Work out the finished part from the listing and answer in its coordinate system (mm). Round coordinates to 2 decimals unless told otherwise and drop trailing zeros. Write each loop counter-clockwise with the first axis right and the second up, starting at its lowest first coordinate (ties: lowest second). Pieces come first, ordered by that corner, then holes. Notation, with made-up numbers: (-1.5, 53) - (47.5, 53) arc R32 ccw to (47.5, 80) - close; hole circle Ø6 at (15.25, 45.5). An arc over 180 degrees is marked (long way). Answer as a JSON object with one key per item and string values.
```python
from build123d import *

# Parameters (mm, degrees)
BOSS_EXTRUDE1_DEPTH = 774.7
SKETCH2_W           = 344.402501539
SKETCH2_H           = 780.457540957
CUT_EXTRUDE1_DEPTH  = 59.371664787


with BuildPart() as part:
    # Sketch1 → Boss-Extrude1 (new body)
    with BuildSketch(Plane(origin=(0, 0, 0), x_dir=(0, 0, -1), z_dir=(1, 0, 0))):
        with BuildLine():
            Line((0, 0), (31.75, 0))
            ThreePointArc((31.75, 0), (54.200640303, 9.299359697), (63.5, 31.75))
            Line((63.5, 31.75), (63.5, 95.25))
            ThreePointArc((63.5, 95.25), (54.200640303, 117.700640303), (31.75, 127))
            Line((31.75, 127), (0, 127))
            Line((0, 127), (-19.05, 127))
            Line((-19.05, 127), (-19.05, 0))
            Line((-19.05, 0), (0, 0))
        make_face()
    extrude(amount=BOSS_EXTRUDE1_DEPTH)

    # Sketch2 → Cut-Extrude1 (cut, through all)
    with BuildSketch(Plane(origin=(355.6, 0, 355.6), x_dir=(0, 1, 0), z_dir=(0.707106781, 0, 0.707106781))):
        with Locations((32.995160032, -592.696903991)):
            Rectangle(SKETCH2_W, SKETCH2_H)
    cut_extrude1 = extrude(amount=CUT_EXTRUDE1_DEPTH, mode=Mode.SUBTRACT)

    # Mirror1: Cut-Extrude1 across plane
    add(cut_extrude1.mirror(Plane(origin=(387.35, 0, 0), x_dir=(0, 0, 1), z_dir=(1, 0, 0))), mode=Mode.SUBTRACT)


solid = part.part
```
Item 1: Each of these flat-tipped pins is pushed along its axis until it touches: P1, Ø12, axis at x = 318.5, z = -42, coming from the +Y side; P2, Ø5, axis at y = 87.5, z = -35.5, coming from the -X side; P3, Ø1.5, axis at x = 325, z = -46.5, coming from the -Y side. Where does it stop, or does it pass through?
Results found:
{"P1": "y = 126.71", "P2": "x = 25.5", "P3": "y = 3.25"}
Item 2: A cutting plane is placed at D-D (x = 57). Write down the section's boundary in (y, z), and give its area (3 significant figures).
Results found:
{"outline": "(0, -31.75) arc R31.75 ccw to (31.75, -63.5) - (95.25, -63.5) arc R31.75 ccw to (127, -31.75) - (127, -6.5) - (0, -6.5) - close", "area": "6,810 mm²"}
Item 3: A cutting plane is placed at A-A (x = 667). Write down the section's boundary in (y, z).
Results found:
{"outline": "(0, -31.75) arc R31.75 ccw to (31.75, -63.5) - (95.25, -63.5) arc R31.75 ccw to (127, -31.75) - (127, 19.05) - (0, 19.05) - close"}
Item 4: A cutting plane is placed at B-B (z = 11). Write down the section's boundary in (x, y).
Results found:
{"outline": "(74.5, 0) - (700.2, 0) - (700.2, 127) - (74.5, 127) - close"}
Item 5: Consider line 1 along X through (y, z) = (21, 4); line 2 along X through (y, z) = (37.5, 12); line 3 along Y through (x, z) = (443, -40). Determine where each line is inside the solid, lowest interval first.
Results found:
{"line 1": "67.5 to 707.2", "line 2": "75.5 to 699.2", "line 3": "1.09 to 125.91"}
Item 6: A cutting plane is placed at C-C (y = 41). Write down the section's boundary in (x, z).
Results found:
{"outline": "(0, -63.5) - (774.7, -63.5) - (692.15, 19.05) - (82.55, 19.05) - close"}
